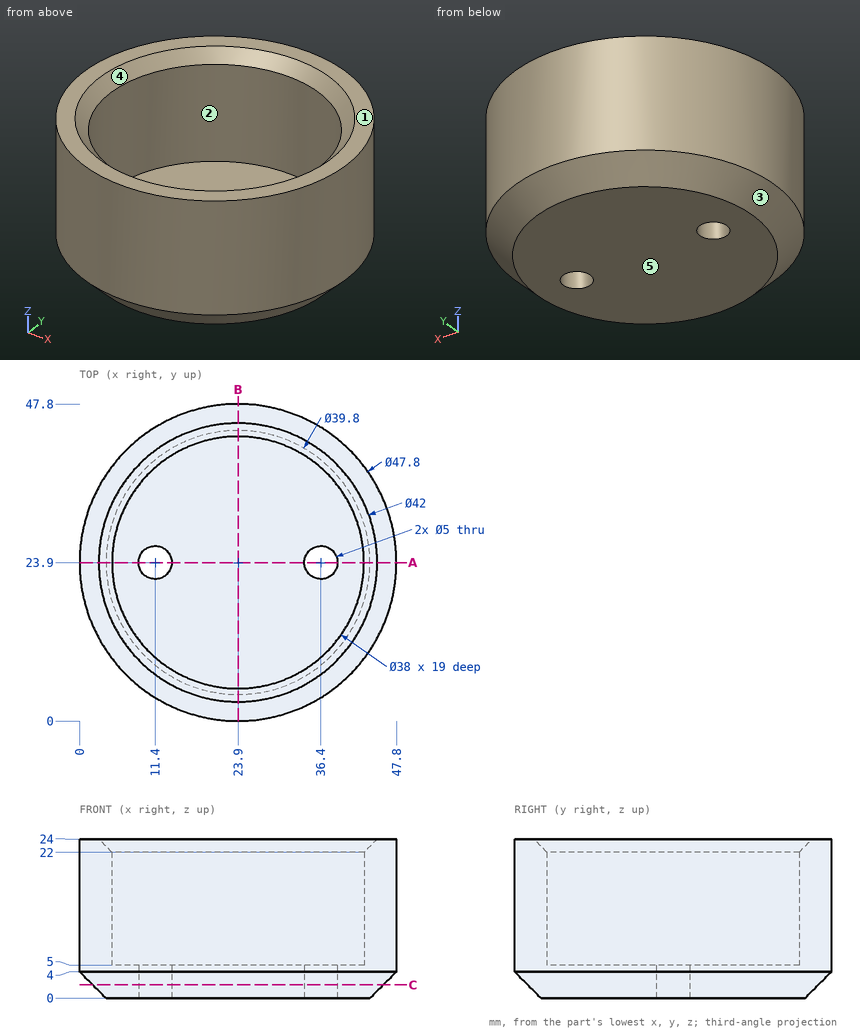
Geometry check sheet. Reference: drawing and pictorial views, mm from the part's lowest x, y, z. A direction names the side the tool comes from. Round coordinates to 2 decimals unless told otherwise and drop trailing zeros. Order: outer loops, then holes, each group sorted by start corner. A loop starts at its lowest first (then second) coordinate and runs counter-clockwise, first axis right, second up.
Q1. Cross-section at B-B, the plane x = 23.9. Enter the section's corners in (y, z).
Filled sheet:
outline: (0, 4) - (4, 0) - (43.8, 0) - (47.8, 4) - (47.8, 24) - (44.9, 24) - (42.9, 22) - (42.9, 5) - (4.9, 5) - (4.9, 22) - (2.9, 24) - (0, 24) - close
Q2. Draft check along X on the marked faces 3, 4 and 5. Enter one of: pulls with the +X half, pulls with the -X half, needs draft (parallel to the pull), parting line crosses it, or undercut.
Filled sheet:
face 3: parting line crosses it
face 4: undercut
face 5: needs draft
Q3. Depth check by flat-ended pin: P1, Ø8, axis at x = 34.5, z = 16.5, coming from the +Y side; P2, Ø5, axis at y = 9, z = 18.5, coming from the -X side; P3, Ø23, axis at x = 23.9, y = 23.9, coming from the +Z side. Enter the tip coordinate at first touch or a pass-through.
Filled sheet:
P1: stops at y = 46.87
P2: stops at x = 3.47
P3: stops at z = 5
Q4. Cross-section at A-A, the plane y = 23.9. Enter the section's corners in (x, z), plus the area to 3 significant figures.
Filled sheet:
outline: (0, 4) - (4, 0) - (8.9, 0) - (8.9, 5) - (4.9, 5) - (4.9, 22) - (2.9, 24) - (0, 24) - close; (13.9, 0) - (33.9, 0) - (33.9, 5) - (13.9, 5) - close; (38.9, 0) - (43.8, 0) - (47.8, 4) - (47.8, 24) - (44.9, 24) - (42.9, 22) - (42.9, 5) - (38.9, 5) - close
area: 355 mm2
Q5. Cross-section at C-C, the plane z = 2. Enter the section's corners in (x, y).
Filled sheet:
outline: circle Ø43.8 at (23.9, 23.9); hole circle Ø5 at (11.4, 23.9); hole circle Ø5 at (36.4, 23.9)
Q6. Set-up check for the marked faces 1 and 2: record each of +Z, -Z, +X, -X, +Y, -Y from which the full face is reachable in a straight line by a thin tool's end or side.
Filled sheet:
face 1: +Z, +X, -X, +Y, -Y
face 2: +Z
Q7. Scan lines: L1, parallel to Y at x = 23.9, z = 8.5; L2, parallel to Z at x = 39.5, y = 20; L3, parallel to Y at x = 36.4, z = 2.4. Record each from-to range of solid material in increasing order.
Filled sheet:
L1: y = 0 to 4.9, 42.9 to 47.8
L2: z = 0 to 5
L3: y = 5.43 to 21.4, 26.4 to 42.37
